Verification items for this drawing (mm, ordinates from the low corner). A direction names the side the tool comes from. Round coordinates to 2 decimals unless told otherwise and drop trailing zeros. Write each loop counter-clockwise with the first axis right and the second up, starting at its lowest first coordinate (ties: lowest second). Pieces come first, ordered by that corner, then holes. Notation, with made-up numbers: (51, -21) -> (66, -21) arc R14 cw to (66, -16) -> close; hole circle Ø1 at (-26.75, 6). An arc over 180 degrees is marked (long way). Return JSON: item names as keys, results as strings. Group by question number.
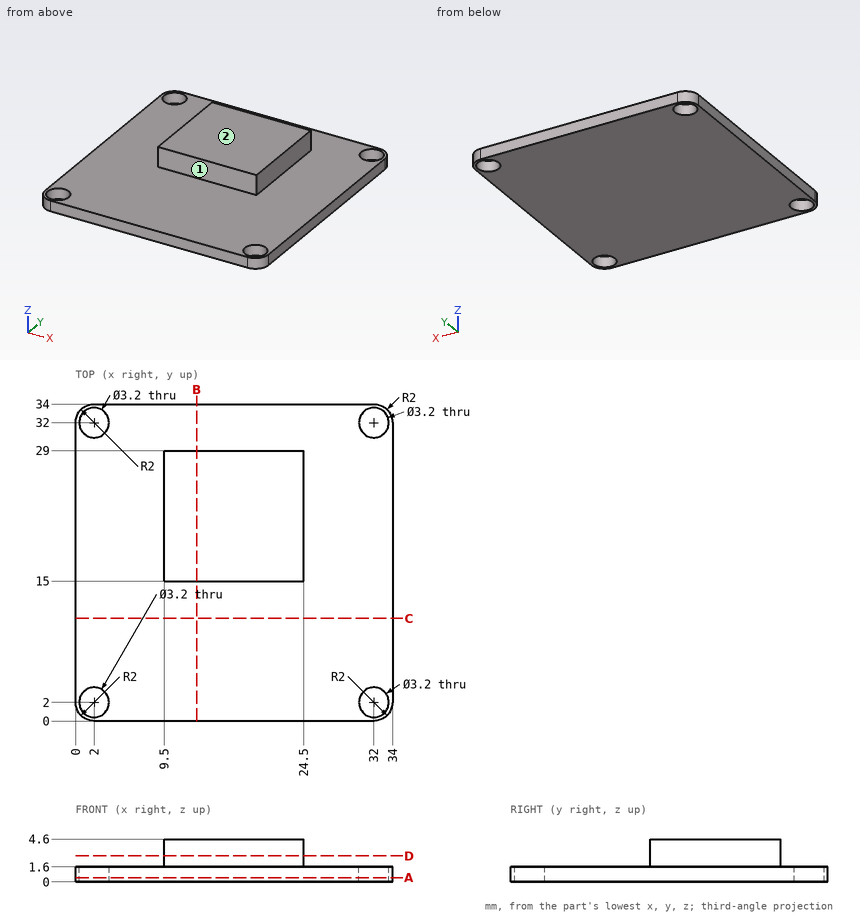
1) Go/stop test with flat-tipped pins: P1, Ø2.5, axis at y = 20, z = 3.5, coming from the +X side; P2, Ø2.5, axis at x = 14.5, z = 3.5, coming from the -Y side; P3, Ø1.9, axis at x = 32, y = 32, coming from the -Z side; P4, Ø4, axis at x = 27, y = 16.5, coming from the +Z side. Record where each tip stops, or that it passes through.
2) Sectioned sample at A-A on z = 0.45. Enter the section's corners in (x, y).
3) Sectioned sample at B-B on x = 13. Enter the section's corners in (y, z).
4) Material ranges on probe 1 along Y at (x, z) = (2.5, 0.4); probe 2 along Y at (x, z) = (32, 0.55); probe 3 along Z at (x, y) = (9, 29.5), recorded low to high. Write a range as [from, to].
5) Tool access check on the marked faces 1 and 2. Record the directions out of +Z, -Z, +X, -X, +Y, -Y that give a thin tool (end or side, any length) a straight path to the whole face; none if there is none.
6) Sectioned sample at D-D on z = 2.8. Enter the section's corners in (x, y), and give its area (3 significant figures).
7) Sectioned sample at C-C on y = 11. Enter the section's corners in (x, z).
Evaluation:
{
 "1": {"P1": "stops at x = 24.5", "P2": "stops at y = 15", "P3": "passes through", "P4": "stops at z = 1.6"},
 "2": {"outline": "(0, 2) arc R2 ccw to (2, 0) -> (32, 0) arc R2 ccw to (34, 2) -> (34, 32) arc R2 ccw to (32, 34) -> (2, 34) arc R2 ccw to (0, 32) -> close; hole circle Ø3.2 at (2, 2); hole circle Ø3.2 at (2, 32); hole circle Ø3.2 at (32, 2); hole circle Ø3.2 at (32, 32)"},
 "3": {"outline": "(0, 0) -> (34, 0) -> (34, 1.6) -> (29, 1.6) -> (29, 4.6) -> (15, 4.6) -> (15, 1.6) -> (0, 1.6) -> close"},
 "4": {"probe 1": "y = [0, 0.48], [3.52, 30.48], [33.52, 34]", "probe 2": "y = [0, 0.4], [3.6, 30.4], [33.6, 34]", "probe 3": "z = [0, 1.6]"},
 "5": {"face 1": "+Z, +X, -X, -Y", "face 2": "+Z, +X, -X, +Y, -Y"},
 "6": {"outline": "(9.5, 15) -> (24.5, 15) -> (24.5, 29) -> (9.5, 29) -> close", "area": "210 mm2"},
 "7": {"outline": "(0, 0) -> (34, 0) -> (34, 1.6) -> (0, 1.6) -> close"}
}
